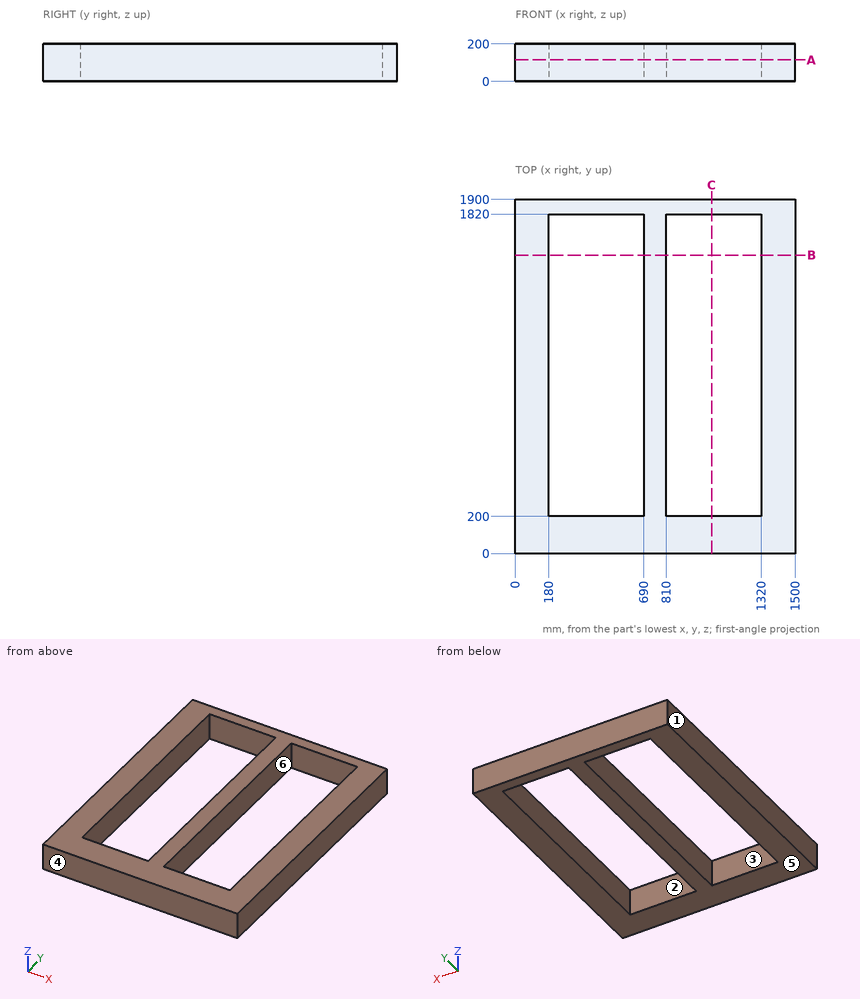
Here's the drawing with two shaded views (mm, measured from the low corner). I have some questions. A direction names the side the tool comes from. Round coordinates to 2 decimals unless told otherwise and drop trailing zeros. Order: outer loops, then holes, each group sorted by start corner. A loop starts at its lowest first (then second) coordinate and runs counter-clockwise, first axis right, second up. Notation, with made-up numbers: (-35.5, 65) -> (-21.5, 65) arc R16 cw to (-21.5, 88) -> close; hole circle Ø11 at (-40, 24). An arc over 180 degrees is marked (long way). Return JSON: item names as keys, results as strings.
Q1. I need wall thicknesses on line 1 along X through (y, z) = (1382, 82.5); line 2 along Y through (x, z) = (298, 60.5). Which ranges of each line are inside material? Lowest first, please. Write a range as from..to.
Filled sheet:
{"line 1": "x = 0..180, 690..810, 1320..1500", "line 2": "y = 0..200, 1820..1900"}
Q2. If we section it at A-A on z = 115.5: List the corners of the cut face in (x, y) for me.
Filled sheet:
{"outline": "(0, 0) -> (1500, 0) -> (1500, 1900) -> (0, 1900) -> close; hole (180, 200) -> (690, 200) -> (690, 1820) -> (180, 1820) -> close; hole (810, 200) -> (1320, 200) -> (1320, 1820) -> (810, 1820) -> close"}
Q3. If we mould it in two halves opening along Y, with no side actions, what happens to the marked faces 1, 2, 3 and 4? For each: released by +Y, released by -Y, zero draft, split by the parting line, or undercut.
Filled sheet:
{"face 1": "zero draft", "face 2": "undercut", "face 3": "undercut", "face 4": "released by -Y"}
Q4. If we section it at B-B on y = 1600: List the corners of the cut face in (x, z) for me, plus the area to 3 significant figures.
Filled sheet:
{"outline": "(0, 0) -> (180, 0) -> (180, 200) -> (0, 200) -> close; (690, 0) -> (810, 0) -> (810, 200) -> (690, 200) -> close; (1320, 0) -> (1500, 0) -> (1500, 200) -> (1320, 200) -> close", "area": "96,000 mm^2"}
Q5. Which directions (+Z, -Z, +X, -X, +Y, -Y) give clear straight access to the entire face, cutting with the end or side of a thin tool? Please do the marked faces 5 and 6.
Filled sheet:
{"face 5": "-Z, +X, -X, +Y, -Y", "face 6": "+Z, -Z"}
Q6. If we section it at C-C on x = 1052.5: List the corners of the cut face in (y, z) for me, plus the area to 3 significant figures.
Filled sheet:
{"outline": "(0, 0) -> (200, 0) -> (200, 200) -> (0, 200) -> close; (1820, 0) -> (1900, 0) -> (1900, 200) -> (1820, 200) -> close", "area": "56,000 mm^2"}
